Work out the finished part from the listing and answer in its coordinate system (mm). A direction names the side the tool comes from. Coordinates: 2 decimals unless noted, no trailing zeros. Loops run counter-clockwise (first coordinate to the right, second up) from the corner with the lowest first, then second, coordinate; pieces in that order, holes last.
```python
from build123d import *

# Parameters (mm, degrees)
BOSS_EXTRUDE1_DEPTH = 3
SKETCH4_W           = 3.2
SKETCH4_H           = 5.925
SKETCH4_W_2         = 23.2
SKETCH4_H_2         = 4.8
SKETCH4_W_3         = 9.1
SKETCH4_W_4         = 5.3
SKETCH4_H_3         = 2.225
CUT_EXTRUDE2_DEPTH  = 4


with BuildPart() as part:
    # Sketch1 → Boss-Extrude1 (new body)
    with BuildSketch(Plane.XY):
        Polygon((21.5, 37.95), (-21.5, 37.95), (-21.5, 15.05), (-8.3, 15.05), (-8.3, 24), (0.7, 24), (0.7, 15.05), (21.5, 15.05), align=None)
    extrude(amount=BOSS_EXTRUDE1_DEPTH)

    # Sketch4 → Cut-Extrude2 (cut, through all)
    with BuildSketch(Plane.XY):
        with Locations((20, 23.6375)):
            Rectangle(SKETCH4_W, SKETCH4_H)
        with Locations((20, 35.0875)):
            Rectangle(SKETCH4_W, SKETCH4_H)
        with Locations((-1.9, 17.35)):
            Rectangle(SKETCH4_W_2, SKETCH4_H_2)
        with Locations((5.15, 35.65)):
            Rectangle(SKETCH4_W_3, SKETCH4_H_2)
        with Locations((-20, 23.6375)):
            Rectangle(SKETCH4_W, SKETCH4_H)
        with Locations((-20, 35.0875)):
            Rectangle(SKETCH4_W, SKETCH4_H)
        with Locations((-10.85, 35.65)):
            Rectangle(SKETCH4_W_4, SKETCH4_H_2)
        with Locations((-3.8, 25.0125)):
            Rectangle(SKETCH4_W, SKETCH4_H_3)
    extrude(amount=CUT_EXTRUDE2_DEPTH, mode=Mode.SUBTRACT)


solid = part.part
```
1. A cutting plane is placed at B-B, the plane y = 19. Give the vertices of the cut face in (x, z).
2. A cutting plane is placed at D-D, the plane x = 6. Give the vertices of the cut face in (y, z), then the cut area to 3 significant figures.
3. Each of these flat-tipped pins is pushed along its axis until it touches: P1, Ø1, axis at y = 24.5, z = 1.5, coming from the -X side; P2, Ø8, axis at x = 16.5, y = 30.5, coming from the -Z side; P3, Ø3, axis at x = -5.5, y = 19, coming from the -Z side; P4, Ø1.5, axis at x = 4.5, z = 1, coming from the +Y side. Where does it stop, or does it pass through?
4. For faces 1 (the flat face through (-4, 26.125, 1)), 2 (the flat face through (-8.2, 36, 1)), 3 (the flat face through (20, 32.125, 1)), 4 (the flat face through (-20, 20.675, 1)), determine the directions among +Z, -Z, +X, -X, +Y, -Y from which every point of the face is accessible in a straight line to the end or side of a thin tool.
5. Straight lines are drawn through the part: probe 1 along X at (y, z) = (34.75, 1.85); probe 2 along X at (y, z) = (21.75, 2.45); probe 3 along X at (y, z) = (24.5, 0.5). For each, find the intervals that lie inside material, in ascending order.
6. A cutting plane is placed at A-A, the plane y = 36. Give the vertices of the cut face in (x, z), then the cut area to 3 significant figures.
7. A cutting plane is placed at C-C, the plane x = -0.5. Give the vertices of the cut face in (y, z), then the cut area to 4 significant figures.
Answers below:
1. outline: (-21.5, 0) - (-13.5, 0) - (-13.5, 3) - (-21.5, 3) - close; (9.7, 0) - (21.5, 0) - (21.5, 3) - (9.7, 3) - close
2. outline: (19.75, 0) - (33.25, 0) - (33.25, 3) - (19.75, 3) - close
2. area: 40.5 mm2
3. P1: stops at x = -18.4
3. P2: stops at z = 0
3. P3: passes through
3. P4: stops at y = 33.25
4. face 1: +Z, -Z, -Y
4. face 2: +Z, -Z, +Y
4. face 3: +Z, -Z, +X, +Y
4. face 4: +Z, -Z, -X
5. probe 1: x = -18.4 to -13.5, -8.2 to 0.6, 9.7 to 18.4
5. probe 2: x = -18.4 to -8.3, 0.7 to 18.4
5. probe 3: x = -18.4 to -5.4, -2.2 to 18.4
6. outline: (-18.4, 0) - (-13.5, 0) - (-13.5, 3) - (-18.4, 3) - close; (-8.2, 0) - (0.6, 0) - (0.6, 3) - (-8.2, 3) - close; (9.7, 0) - (18.4, 0) - (18.4, 3) - (9.7, 3) - close
6. area: 67.2 mm2
7. outline: (24, 0) - (37.95, 0) - (37.95, 3) - (24, 3) - close
7. area: 41.85 mm2
